Autodesk Fusion 360 part; units mm, degrees
sketch "スケッチ1" plane through (0, 0, 0) normal (0, 0, 1) x (1, 0, 0)
  line L0 (0, 0) -> (2.54, 0)
  line L1 (2.54, 0) -> (2.54, 2.54)
  line L2 (2.54, 2.54) -> (0, 2.54)
  line L3 (0, 2.54) -> (0, 0)
  circle A0 centre (1.27, 1.27) radius 0.3
  dimension "d1" = 2.54
  dimension "d2" = 2.54
  dimension "d12" = 0.6
  dimension "d13" = 1.27
  dimension "d14" = 1.27
extrude "押し出し1" add sketch "スケッチ1" along normal blind 2.7 contours L0 L1 L2 L3 | A0
sketch "スケッチ2" plane through (0, 0, 2.7) normal (0, 0, 1) x (-1, 0, 0)
  line L0 (0, -2.54) -> (0, 0)
  line L1 (0, 0) -> (-2.54, 0)
  line L2 (-2.54, 0) -> (-2.54, -2.54)
  line L3 (-2.54, -2.54) -> (0, -2.54)
  line L4 (-0.97, -1.57) -> (-1.57, -1.57)
  line L5 (-1.57, -1.57) -> (-1.57, -0.97)
  line L6 (-1.57, -0.97) -> (-0.97, -0.97)
  line L7 (-0.97, -0.97) -> (-0.97, -1.57)
  dimension "d5" = 0.6
  dimension "d6" = 0.6
  dimension "d7" = 0.97
  dimension "d8" = 0.97
extrude "押し出し2" add sketch "スケッチ2" along normal blind 5.7 contours L4 L5 L6 L7
chamfer "面取り1" distance 0.2 angle 45 4 edges at (1.27, 0.97, 8.4) (1.57, 1.27, 8.4) (1.27, 1.57, 8.4) (0.97, 1.27, 8.4)
extrude "押し出し3" add sketch "スケッチ1" against normal blind 3 contours A0
chamfer "面取り2" distance 0.3 angle 45 4 edges at (0, 2.54, 1.35) (0, 0, 1.35) (2.54, 0, 1.35) (2.54, 2.54, 1.35)
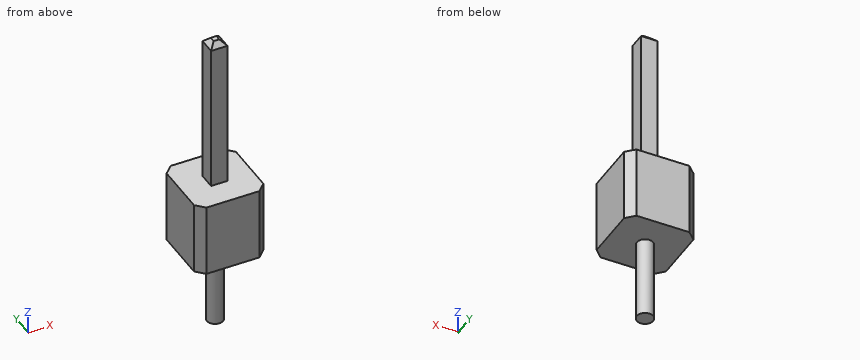
Model file for the job. Use its own axes, mm. Give positions to 0.01 mm unless a question says otherwise; leave off trailing zeros. Write each loop counter-clockwise with the first axis right and the second up, starting at its lowest first coordinate (ties: lowest second). Pieces come first, ordered by that corner, then holes. Notation, with made-up numbers: M 28.5,-26 L 59.5,-26 A30 ccw 59.5,-2 Z; hole C 73,38.5 d8. An arc over 180 degrees is marked long. One line per item, written item: value. Start each with the question number.
Q1. Saw through at A-A, the plane x = 1.27. Write the cut outline in (y, z), plus the area to 3 significant figures.
Q2. Saw through at D-D, the plane z = 3.75. Write the cut outline in (x, y), plus the area to 3 significant figures.
Q3. Probe probe 1 along Z at (x, y) = (2.35, 1.85); probe 2 along X at (y, z) = (1.15, 6). List the from-to ranges inside material, lowest first. Write a range as [from, to].
Q4. Drop flat-ended pins along their axis: pin 1 Ø0.7 at (x, z) = (1, 6) entering from +Y; pin 2 Ø0.5 at (y, z) = (1.5, 5.5) entering from -X; pin 3 Ø0.8 at (x, y) = (2, 1) entering from +Z. Give the stop position or say it passes through.
Q5. Saw through at B-B, the plane z = 0.5. Write the cut outline in (x, y), plus the area to 3 significant figures.
Output values:
1. outline: M 0,0 L 0.97,0 L 0.97,-3 L 1.57,-3 L 1.57,0 L 2.54,0 L 2.54,2.7 L 1.57,2.7 L 1.57,8.2 L 1.37,8.4 L 1.17,8.4 L 0.97,8.2 L 0.97,2.7 L 0,2.7 Z
1. area: 12.0 mm²
2. outline: M 0.97,0.97 L 1.57,0.97 L 1.57,1.57 L 0.97,1.57 Z
2. area: 0.360 mm²
3. probe 1: z = [0, 2.7]
3. probe 2: x = [0.97, 1.57]
4. pin 1: stops at y = 1.57
4. pin 2: stops at x = 0.97
4. pin 3: stops at z = 2.7
5. outline: M 0,0.3 L 0.3,0 L 2.24,0 L 2.54,0.3 L 2.54,2.24 L 2.24,2.54 L 0.3,2.54 L 0,2.24 Z
5. area: 6.27 mm²
